Can you work these out from the drawing? Everything is in mm from the part's minimum corner. A direction names the side the tool comes from. Give positions to 0.01 mm unless a question says otherwise; leave off trailing zeros. Loops run counter-clockwise (first coordinate to the right, second up) from the corner with the lowest first, then second, coordinate; pieces in that order, holes last. Notation, with made-up numbers: M 88.5,35.25 L 93.5,35.25 A21 cw 93.5,67.25 Z; hole C 36,56.5 d2. An arc over 180 degrees is marked long. Use CSV: the item, a comma, the result in double quotes.
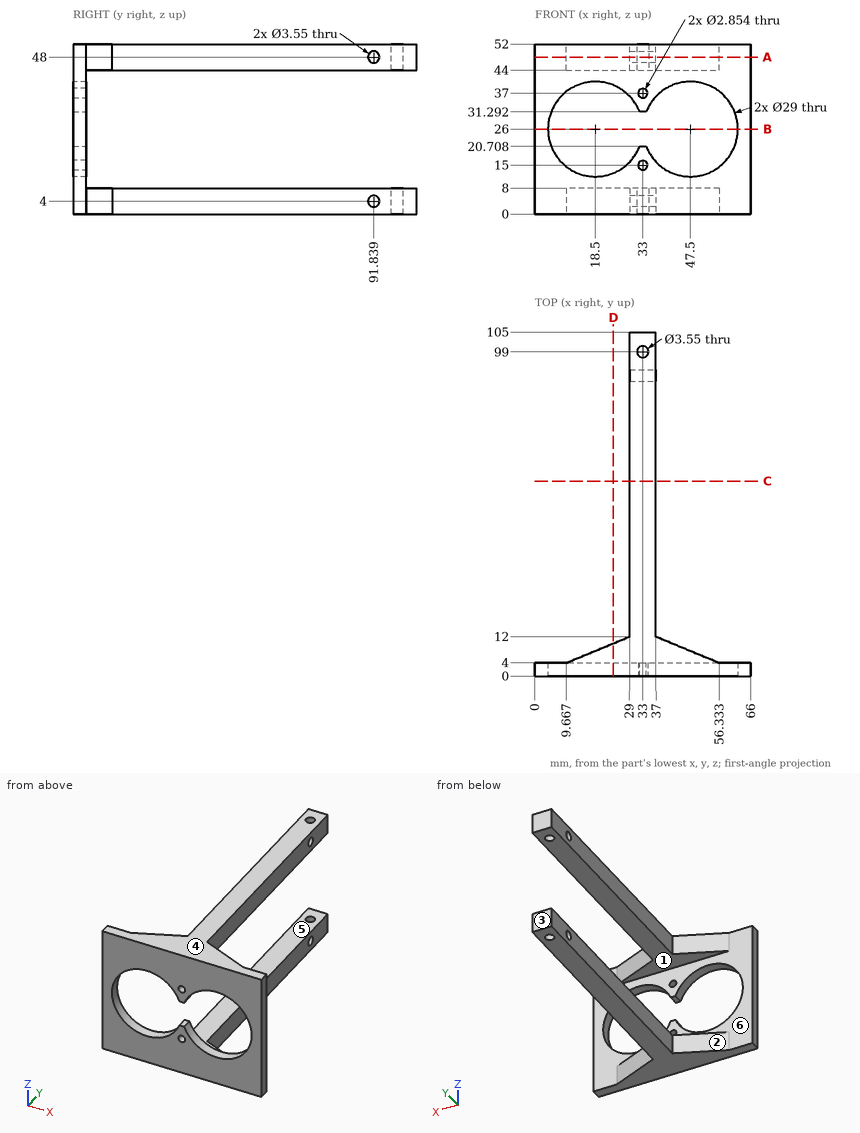
Q1. I want a section at C-C, the plane y = 59.5. Please give me the cut outline in (x, z).
Model answer:
outline,"M 29,0 L 37,0 L 37,8 L 29,8 Z; M 29,44 L 37,44 L 37,52 L 29,52 Z"
Q2. If we mould it in two halves opening along Z, with no side actions, what happens to the marked faces 3, 4, 5 and 6? For each: released by +Z, released by -Z, zero draft, split by the parting line, or undercut.
Model answer:
face 3,"zero draft"
face 4,"released by +Z"
face 5,"undercut"
face 6,"undercut"
Q3. For the marked faces 1 and 2, which set-ups out of +Z, -Z, +X, -X, +Y, -Y let a thin tool reach every point of the face, with its end or its side?
Model answer:
face 1,"+X, -X, +Y"
face 2,"+Z, -Z, -X, +Y"
Q4. I want a section at D-D, the plane x = 24. Please give me the cut outline in (y, z).
Model answer:
outline,"M 0,0 L 9.93,0 L 9.93,8 L 4,8 L 4,12.58 L 0,12.58 Z; M 0,39.42 L 4,39.42 L 4,44 L 9.93,44 L 9.93,52 L 0,52 Z"
Q5. I want a section at B-B, the plane z = 26. Please give me the cut outline in (x, y), then the cut area to 3 significant figures.
Model answer:
outline,"M 0,0 L 4,0 L 4,4 L 0,4 Z; M 62,0 L 66,0 L 66,4 L 62,4 Z"
area,"32.0 mm2"
Q6. I'm going to push flat-ended pins straight in: P1, Ø6.5, axis at y = 63, z = 3.5, coming from the +X side; P2, Ø6, axis at x = 49, z = 44, coming from the +Y side (1 decimal); P3, Ø5, axis at x = 25.5, y = 12.5, coming from the -Z side; P4, Ø6.5, axis at y = 55, z = 46.5, coming from the -X side. Where does each tip first touch, or does it pass through?
Model answer:
P1,"x = 37"
P2,"y = 8.3"
P3,"z = 0"
P4,"x = 29"
Q7. Please list where these lines run through material, in increasing order: L1, parallel to Y at x = 34.25, z = 4 (1 decimal); L2, parallel to Y at x = 33, z = 50 (1 decimal); L3, parallel to Z at x = 18.5, y = 2.3. Write a range as from..to.
Model answer:
L1,"0..90.1, 93.6..97.7, 100.3..105"
L2,"0..97.2, 100.8..105"
L3,"0..11.5, 40.5..52"
Q8. I want a section at A-A, the plane z = 48. State how many separate pieces and enclosed holes the cut face has, then the cut area to 3 significant figures.
Model answer:
separate pieces,"2"
enclosed holes,"1"
area,"1,190 mm2"
